Input: dimensioned drawing with shaded views. Units: mm. Origin: part minimum x, y, z. Coordinates: 2 decimals unless noted, no trailing zeros. Order: outer loops, then holes, each group sorted by start corner. A loop starts at its lowest first (then second) coordinate and runs counter-clockwise, first axis right, second up. Notation, with made-up numbers: (-31, -31.75) -> (-5, -31.75) arc R22 ccw to (-5, 4.25) -> close; hole circle Ø7 at (-4, 15). An arc over 180 degrees is marked (long way). Answer in a Markdown table with one row per item. Add a question column.
1) Contact query for flat-ended pins moving along their axis: P1, Ø3, axis at x = 679, z = 253.5, coming from the -Y side; P2, Ø1, axis at x = 408, y = 30.5, coming from the +Z side; P3, Ø11, axis at y = 50.5, z = 282.5, coming from the -X side. Output: stop coordinate, or through.
2) Ray query, line 1 (X direction, y = 31.75, z = 282); line 2 (Y direction, x = 381, z = 283); line 3 (X direction, y = 31, z = 285). Return the intervals inside material, ascending. Write a range as from..to.
3) Section query C-C on x = 268. Return the cut outline in (y, z).
4) Section query B-B on z = 69. Return the cut outline in (x, y).
5) Section query A-A on x = 381. Return the cut outline in (y, z).
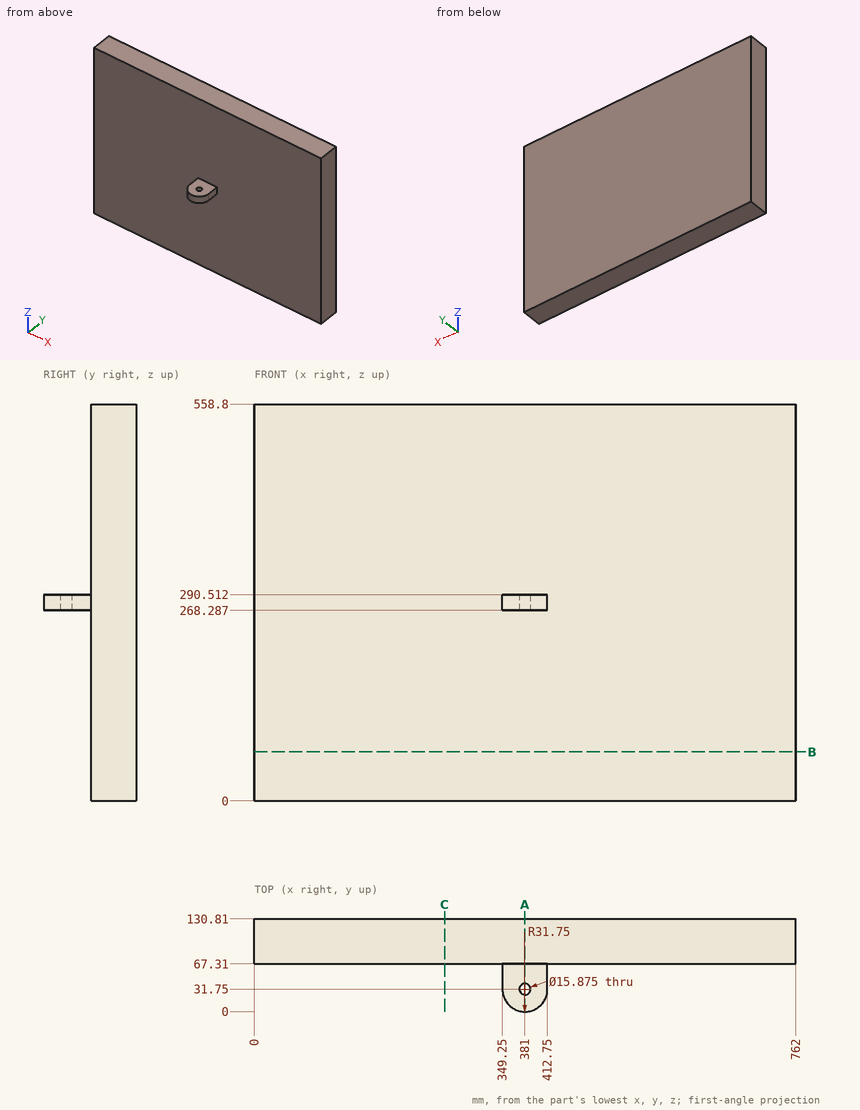
Result:
| question | item | result |
|---|---|---|
| 1 | P1 | y = 67.31 |
| 1 | P2 | z = 290.51 |
| 1 | P3 | x = 349.25 |
| 2 | line 1 | 349.25..373.06, 388.94..412.75 |
| 2 | line 2 | 0..23.81, 39.69..130.81 |
| 2 | line 3 | 349.26..373.1, 388.9..412.74 |
| 3 | outline | (67.31, 0) -> (130.81, 0) -> (130.81, 558.8) -> (67.31, 558.8) -> close |
| 4 | outline | (0, 67.31) -> (762, 67.31) -> (762, 130.81) -> (0, 130.81) -> close |
| 5 | outline | (0, 268.29) -> (23.81, 268.29) -> (23.81, 290.51) -> (0, 290.51) -> close; (39.69, 268.29) -> (67.31, 268.29) -> (67.31, 0) -> (130.81, 0) -> (130.81, 558.8) -> (67.31, 558.8) -> (67.31, 290.51) -> (39.69, 290.51) -> close |
